```python
from build123d import *

# Parameters (mm, degrees)
SKETCH1_W           = 13
SKETCH1_H           = 5
BOSS_EXTRUDE1_DEPTH = 11
CUT_EXTRUDE1_DEPTH  = 6
SKETCH3_R           = 0.3
BOSS_EXTRUDE2_DEPTH = 1
FILLET1_R           = 0.2


with BuildPart() as part:
    # Sketch1 → Boss-Extrude1 (new body)
    with BuildSketch(Plane(origin=(0, 0, 0), x_dir=(1, 0, 0), z_dir=(0, 1, 0))):
        Rectangle(SKETCH1_W, SKETCH1_H)
    extrude(amount=BOSS_EXTRUDE1_DEPTH)

    # Sketch2 → Cut-Extrude1 (cut, through all)
    with BuildSketch(Plane.XY.offset(2.5)):
        Polygon((-4.5, 0), (-4, 0.5), (4, 0.5), (4.5, 0), (4.5, -1.5), (-4.5, -1.5), align=None)
    extrude(amount=-CUT_EXTRUDE1_DEPTH, mode=Mode.SUBTRACT)

    # Sketch3 → Boss-Extrude2 (add)
    with BuildSketch(Plane.XZ):
        with Locations((5, 0)):
            Circle(SKETCH3_R)
        with Locations((-5, 0)):
            Circle(SKETCH3_R)
    extrude(amount=BOSS_EXTRUDE2_DEPTH)

    # Fillet1
    fillet1_edges = [part.edges().sort_by_distance(p)[0] for p in [
        (6.5, 11, 0),
        (0, 11, -2.5),
        (-5.5, 0, -2.5),
        (5.5, 0, 2.5),
        (4.25, 0.25, 2.5),
        (0, 0.5, 2.5),
        (-4.25, 0.25, 2.5),
        (-4.25, 0.25, -2.5),
        (-4.5, 0, 0),
        (0, 0.5, -2.5),
        (-4, 0.5, 0),
        (4.25, 0.25, -2.5),
        (4, 0.5, 0),
        (4.5, 0, 0),
        (-6.5, 11, 0),
        (5.5, 0, -2.5),
        (6.5, 0, 0),
        (-5.5, 0, 2.5),
        (-6.5, 0, 0),
        (0, 11, 2.5),
        (-6.5, 5.5, -2.5),
        (6.5, 5.5, -2.5),
        (6.5, 5.5, 2.5),
        (-6.5, 5.5, 2.5),
    ]]
    fillet(fillet1_edges, radius=FILLET1_R)


solid = part.part
```
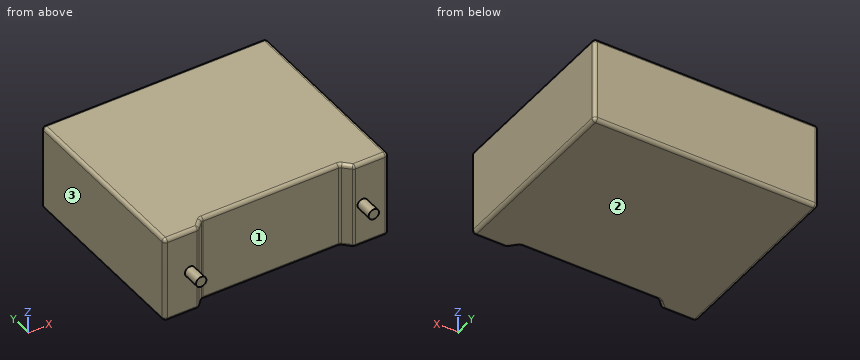
Source: CAD feature listing. Evaluate the final solid. Frame: model axes, mm. Face numbers are marked on the shaded views. Give positions to 0.01 mm unless a question says otherwise; leave off trailing zeros. Write each loop counter-clockwise with the first axis right and the second up, starting at its lowest first coordinate (ties: lowest second). Pieces come first, ordered by that corner, then holes.
1. First-contact query: pin 1 (1.9 mm diameter, centred on x = 5.5, z = 1, fed in from -Y). Flat tip, straight axial feed; report the tip coordinate or a pass-through.
2. Material intervals for line 1 along X through (y, z) = (0.25, 1.1); line 2 along Y through (x, z) = (4.75, 1.7); line 3 along Y through (x, z) = (3, -2.05), sorted ascending.
3. Section query A-A (x = -5). Return the cut outline in (y, z).
4. Section query B-B (z = -1.4). Return the cut outline in (x, y), then the cut area to 3 significant figures.
5. Pull-direction query (X, two-part tool) for the marked faces 1, 2 and 3; classes: +X half, -X half, draft (parallel to the pull), parting line (faces both ways), or undercut.
6. Section query C-C (z = 0). Return the cut outline in (x, y).
7. Section query D-D (x = -2.25). Return the cut outline in (y, z), then the cut area to 3 significant figures.
Output values:
1. pin 1: stops at y = -1
2. line 1: x = -6.5 to -4.25, 4.25 to 6.5
2. line 2: y = 0 to 11
2. line 3: y = 0.5 to 11
3. outline: (-1, -0.3) - (0, -0.3) - (0, -2.3) arc R0.2 ccw to (0.2, -2.5) - (10.8, -2.5) arc R0.2 ccw to (11, -2.3) - (11, 2.3) arc R0.2 ccw to (10.8, 2.5) - (0.2, 2.5) arc R0.2 ccw to (0, 2.3) - (0, 0.3) - (-1, 0.3) - close
4. outline: (-6.5, 0.2) arc R0.2 ccw to (-6.3, 0) - (-4.58, 0) arc R0.2 ccw to (-4.44, 0.06) - (-4.06, 0.44) arc R0.2 cw to (-3.92, 0.5) - (3.92, 0.5) arc R0.2 cw to (4.06, 0.44) - (4.44, 0.06) arc R0.2 ccw to (4.58, 0) - (6.3, 0) arc R0.2 ccw to (6.5, 0.2) - (6.5, 10.8) arc R0.2 ccw to (6.3, 11) - (-6.3, 11) arc R0.2 ccw to (-6.5, 10.8) - close
4. area: 139 mm2
5. face 1: undercut
5. face 2: draft
5. face 3: -X half
6. outline: (-6.5, 0.2) arc R0.2 ccw to (-6.3, 0) - (-5.3, 0) - (-5.3, -1) - (-4.7, -1) - (-4.7, 0) - (-4.58, 0) arc R0.2 ccw to (-4.44, 0.06) - (-4.06, 0.44) arc R0.2 cw to (-3.92, 0.5) - (3.92, 0.5) arc R0.2 cw to (4.06, 0.44) - (4.44, 0.06) arc R0.2 ccw to (4.58, 0) - (4.7, 0) - (4.7, -1) - (5.3, -1) - (5.3, 0) - (6.3, 0) arc R0.2 ccw to (6.5, 0.2) - (6.5, 10.8) arc R0.2 ccw to (6.3, 11) - (-6.3, 11) arc R0.2 ccw to (-6.5, 10.8) - close
7. outline: (0.5, -2.3) arc R0.2 ccw to (0.7, -2.5) - (10.8, -2.5) arc R0.2 ccw to (11, -2.3) - (11, 2.3) arc R0.2 ccw to (10.8, 2.5) - (0.7, 2.5) arc R0.2 ccw to (0.5, 2.3) - close
7. area: 52.5 mm2
